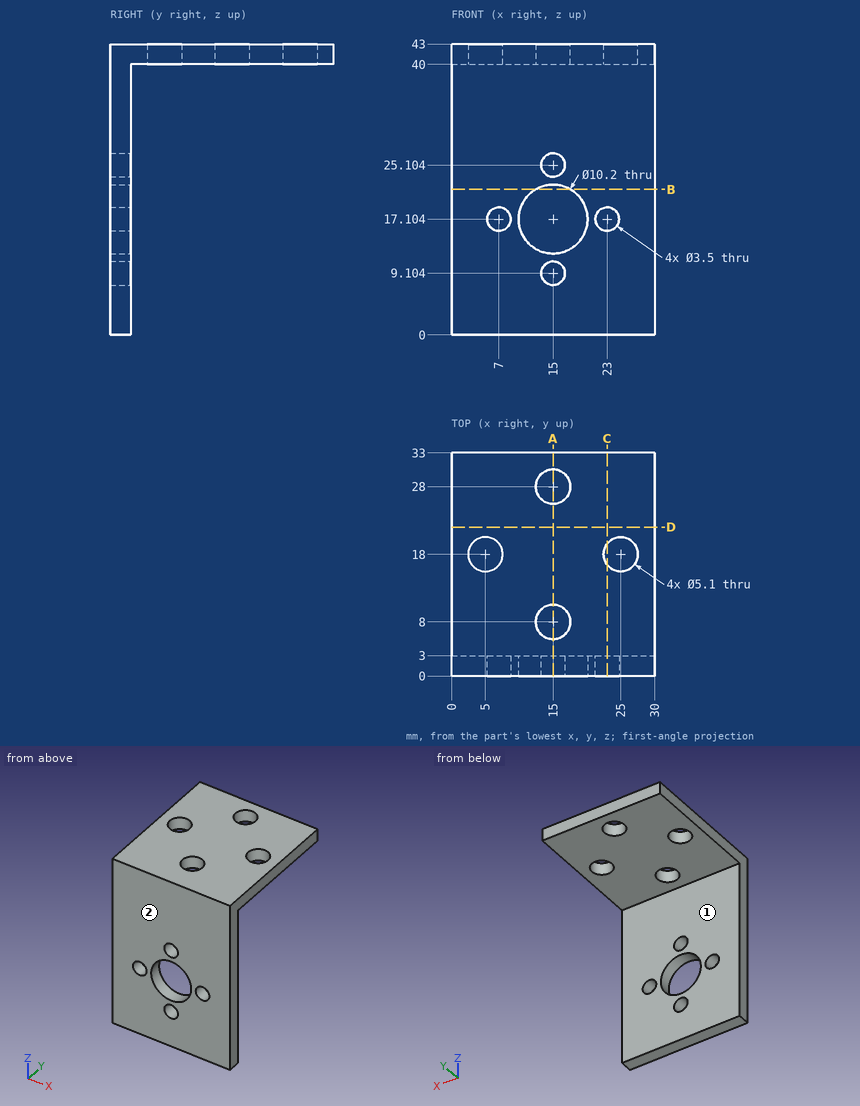
Source: three-view drawing plus pictorial views. Frame: mm from the lowest corner of the part. A direction names the side the tool comes from. Round coordinates to 2 decimals unless told otherwise and drop trailing zeros. Loops run counter-clockwise (first coordinate to the right, second up) from the corner with the lowest first, then second, coordinate; pieces in that order, holes last. Notation, with made-up numbers: (45, -8.5) -> (84, -8.5) arc R13 cw to (84, 7.5) -> close; hole circle Ø11 at (12.25, -16). An arc over 180 degrees is marked (long way). Use one line per item in the form item = value.
Item 1: Cut plane D-D on y = 22. Output: boundary loops of the cut face in (x, z).
Evaluation:
outline = (0, 40) -> (30, 40) -> (30, 43) -> (0, 43) -> close
Item 2: Access query for the marked faces 1 and 2. Directions: +Z, -Z, +X, -X, +Y, -Y. A direction counts if a zero-diameter tool reaches every point of the face in a straight line with its end or side. Return the directions, or none.
Evaluation:
face_1 = -Z, +X, -X, +Y
face_2 = +Z, -Z, +X, -X, -Y
Item 3: Cut plane C-C on x = 23. Output: boundary loops of the cut face in (y, z), then the cut area to 3 significant figures.
Evaluation:
outline = (0, 0) -> (3, 0) -> (3, 15.35) -> (0, 15.35) -> close; (0, 18.85) -> (3, 18.85) -> (3, 40) -> (16.42, 40) -> (16.42, 43) -> (0, 43) -> close; (19.58, 40) -> (33, 40) -> (33, 43) -> (19.58, 43) -> close
area = 199 mm2
Item 4: Material intervals for probe 1 along Y at (x, z) = (15, 41.6); probe 2 along Z at (x, y) = (23, 1.25); probe 3 along Y at (x, z) = (12.5, 29), sorted ascending.
Evaluation:
probe_1 = 0 to 5.45, 10.55 to 25.45, 30.55 to 33
probe_2 = 0 to 15.35, 18.85 to 43
probe_3 = 0 to 3
Item 5: Cut plane A-A on x = 15. Output: boundary loops of the cut face in (y, z).
Evaluation:
outline = (0, 0) -> (3, 0) -> (3, 7.35) -> (0, 7.35) -> close; (0, 10.85) -> (3, 10.85) -> (3, 12) -> (0, 12) -> close; (0, 22.2) -> (3, 22.2) -> (3, 23.35) -> (0, 23.35) -> close; (0, 26.85) -> (3, 26.85) -> (3, 40) -> (5.45, 40) -> (5.45, 43) -> (0, 43) -> close; (10.55, 40) -> (25.45, 40) -> (25.45, 43) -> (10.55, 43) -> close; (30.55, 40) -> (33, 40) -> (33, 43) -> (30.55, 43) -> close
Item 6: Contact query for flat-ended pins moving along their axis: pin 1 Ø4.5 at (x, z) = (7, 17.104) entering from +Y; pin 2 Ø6 at (x, y) = (5, 18) entering from -Z; pin 3 Ø4.5 at (x, z) = (15, 9.104) entering from -Y; pin 4 Ø3 at (x, y) = (25, 18) entering from +Z. Output: stop coordinate, or through.
Evaluation:
pin_1 = 3
pin_2 = 40
pin_3 = 0
pin_4 = through
Item 7: Cut plane B-B on z = 21.5. Output: boundary loops of the cut face in (x, y), then the cut area to 3 significant figures.
Evaluation:
outline = (0, 0) -> (12.41, 0) -> (12.41, 3) -> (0, 3) -> close; (17.59, 0) -> (30, 0) -> (30, 3) -> (17.59, 3) -> close
area = 74.5 mm2
